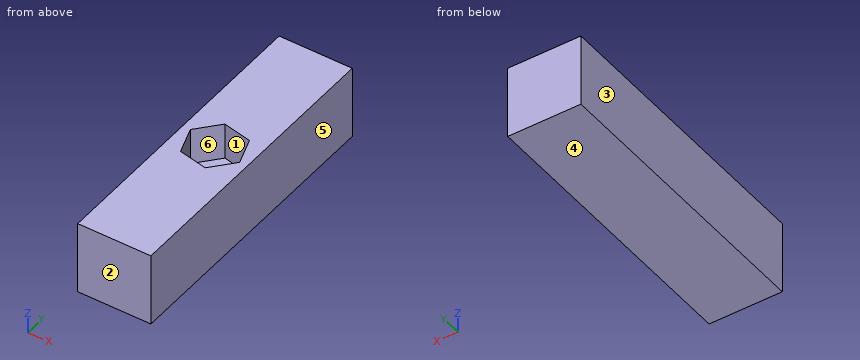
Autodesk Fusion 360 part; units mm, degrees
sketch "Sketch1" plane through (0, 0, 0) normal (0, 0, 1) x (1, 0, 0)
  line L0 (0, 0) -> (10, 0)
  line L1 (10, 0) -> (10, -40)
  line L2 (10, -40) -> (0, -40)
  line L3 (0, -40) -> (0, 0)
  dimension "d1" = 40
  dimension "d2" = 10
extrude "Extrude1" add sketch "Sketch1" along normal blind 10
sketch "Sketch2" plane through (0, 0, 10) normal (0, 0, 1) x (-1, 0, 0)
  line L0 (0, 40) -> (-10, 40)
  line L1 (-10, 40) -> (-10, 0)
  line L2 (-10, 0) -> (0, 0)
  line L3 (0, 0) -> (0, 40)
  line L4 (-6.2649, 23.7947) -> (-8.9188, 20.8019)
  line L5 (-8.9188, 20.8019) -> (-7.6539, 17.0072)
  line L6 (-7.6539, 17.0072) -> (-3.7351, 16.2053)
  line L7 (-3.7351, 16.2053) -> (-1.0812, 19.1981)
  line L8 (-1.0812, 19.1981) -> (-2.3461, 22.9928)
  line L9 (-2.3461, 22.9928) -> (-6.2649, 23.7947)
  point P0 (-5, 20)
  dimension "d5" = 4
extrude "Extrude2" cut sketch "Sketch2" against normal blind 5 contours L4 L5 L6 L7 L8 L9
For this review, take the finished solid that the model builds, in its own axes (mm). Face numbers are marked on the shaded views. A direction names the side the tool comes from. Round coordinates to 2 decimals unless told otherwise and drop trailing zeros. Write each loop counter-clockwise with the first axis right and the second up, starting at its lowest first coordinate (ties: lowest second). Pieces come first, ordered by that corner, then holes. Notation, with made-up numbers: (14, 26.5) - (33, 26.5) arc R25 cw to (33, 42.5) - close; hole circle Ø3 at (-39, -10). An arc over 180 degrees is marked (long way). Answer as a JSON object with one key per item and string values.
1. For pin 1 Ø5 at (x, z) = (8.5, 5.5) entering from +Y, flat-tipped, find the tip position at first contact; note if it passes through.
Response values:
{"pin 1": "stops at y = 0"}
2. Tool access review of the marked faces 1 and 2: name each direction out of +Z, -Z, +X, -X, +Y, -Y from which nothing blocks a thin tool from reaching the whole face with its end or side.
Response values:
{"face 1": "+Z", "face 2": "+Z, -Z, +X, -X, -Y"}
3. We need section B-B on x = 1.5. Give the boundary of the cut face in (y, z).
Response values:
{"outline": "(-40, 0) - (0, 0) - (0, 10) - (-18.73, 10) - (-18.73, 5) - (-20.45, 5) - (-20.45, 10) - (-40, 10) - close"}
4. We need section A-A on z = 9.25. Give the boundary of the cut face in (x, y), then the cut area to 3 significant figures.
Response values:
{"outline": "(0, -40) - (10, -40) - (10, 0) - (0, 0) - close; hole (1.08, -19.2) - (2.35, -22.99) - (6.26, -23.79) - (8.92, -20.8) - (7.65, -17.01) - (3.74, -16.21) - close", "area": "358 mm2"}
5. We need section C-C on y = -18.5. Give the boundary of the cut face in (x, z), then the cut area to 3 significant figures.
Response values:
{"outline": "(0, 0) - (10, 0) - (10, 10) - (8.15, 10) - (8.15, 5) - (1.7, 5) - (1.7, 10) - (0, 10) - close", "area": "67.7 mm2"}
6. Draft analysis for pull direction X (two halves, no side actions). For the marked faces 3, 4, 5 and 6, state which applies: +X half, -X half, draft (parallel to the pull), parting line (faces both ways), or undercut.
Response values:
{"face 3": "-X half", "face 4": "draft", "face 5": "+X half", "face 6": "undercut"}
7. To check wall thickness, follow line 1 along Y through (x, z) = (5.5, 7.25); line 2 along X through (y, z) = (-19, 9); line 3 along X through (y, z) = (-20.5, 6). State the ranges of each line that lie inside material, in increasing order.
Response values:
{"line 1": "y = -40 to -23.64, -16.57 to 0", "line 2": "x = 0 to 1.26, 8.32 to 10", "line 3": "x = 0 to 1.52, 8.82 to 10"}
